Build history of the part. All positions in model axes, mm. Face numbers are marked on the shaded views. A direction names the side the tool comes from. Coordinates: 2 decimals unless noted, no trailing zeros. Loops run counter-clockwise (first coordinate to the right, second up) from the corner with the lowest first, then second, coordinate; pieces in that order, holes last. Notation, with made-up numbers: (53.25, 58.25) - (78.25, 58.25) arc R28 cw to (78.25, 97.25) - close; hole circle Ø5 at (9, 74.25). An arc over 180 degrees is marked (long way). One line per item, written item: value.
```python
from build123d import *

# Parameters (mm, degrees)
SKETCH1_R           = 1.4
BOSS_EXTRUDE1_DEPTH = 8.5


with BuildPart() as part:
    # Sketch1 → Boss-Extrude1 (new body)
    with BuildSketch(Plane(origin=(0, -3.71400402, 0), x_dir=(1, 0, 0), z_dir=(0, 1, 0))):
        with BuildLine():
            ThreePointArc((-114.649243174, 10.730908874), (-116.044111605, 12.812074413), (-118.499243174, 12.312838076))
            Line((-118.499243174, 12.312838076), (-118.499243174, 11.190908874))
            Line((-118.499243174, 11.190908874), (-119.101719053, 11.190908874))
            ThreePointArc((-119.101719053, 11.190908874), (-117.130467384, 8.49282144), (-114.649243174, 10.730908874))
        make_face()
        with Locations((-116.899243174, 10.730908874)):
            Circle(SKETCH1_R, mode=Mode.SUBTRACT)
    extrude(amount=BOSS_EXTRUDE1_DEPTH)


solid = part.part
```
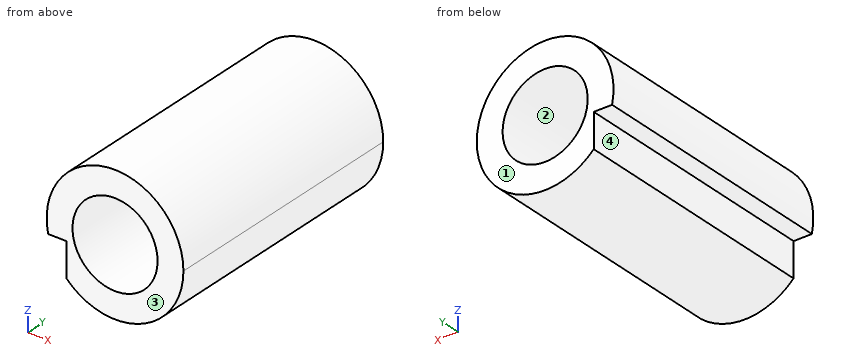
Item 1: Cut at D-D, the plane x = -115.05. Write the cut outline in (y, z).
Check result:
outline: (-3.71, -12.01) - (4.79, -12.01) - (4.79, -9.45) - (-3.71, -9.45) - close
Item 2: Drop flat-ended pins along their axis: P1, Ø0.5, axis at x = -119, y = 1, coming from the -Z side; P2, Ø0.6, axis at y = 1.5, z = -12, coming from the -X side; P3, Ø2, axis at x = -116.9, z = -10.73, coming from the +Y side; P4, Ø1, axis at y = 2, z = -9.5, coming from the -X side. Give the stop position or say it passes through.
Check result:
P1: stops at z = -11.19
P2: stops at x = -118.5
P3: passes through
P4: stops at x = -119.03
Item 3: Cut at A-A, the plane x = -115.8. Write the cut outline in (y, z).
Check result:
outline: (-3.71, -12.69) - (4.79, -12.69) - (4.79, -11.6) - (-3.71, -11.6) - close; (-3.71, -9.86) - (4.79, -9.86) - (4.79, -8.77) - (-3.71, -8.77) - close
Item 4: Pull direction Z, two halves, no side cores. Call the marked faces 1 and 2: released by +Z, released by -Z, zero draft, split by the parting line, or undercut.
Check result:
face 1: zero draft
face 2: undercut
Item 5: Tool access for the marked faces 3 and 4: list every direction of +Z, -Z, +X, -X, +Y, -Y with a clear straight run to the whole face (end or side of a thin tool).
Check result:
face 3: +Z, -Z, +X, -X, -Y
face 4: -Z, -X, +Y, -Y
Item 6: Probe probe 1 along X at (y, z) = (-0.75, -10.75); probe 2 along X at (y, z) = (4.25, -10.25); probe 3 along Z at (x, y) = (-116.4, 1.5). List the from-to ranges inside material, lowest first. Write a range as from..to.
Check result:
probe 1: x = -119.15..-118.3, -115.5..-114.65
probe 2: x = -119.1..-118.21, -115.58..-114.7
probe 3: z = -12.92..-12.04, -9.42..-8.54
Item 7: Cut at B-B, the plane z = -10.4. Write the cut outline in (x, y), then the cut area to 3 significant figures.
Check result:
outline: (-119.12, -3.71) - (-118.26, -3.71) - (-118.26, 4.79) - (-119.12, 4.79) - close; (-115.54, -3.71) - (-114.67, -3.71) - (-114.67, 4.79) - (-115.54, 4.79) - close
area: 14.7 mm^2
Item 8: Cut at C-C, the plane y = 0.25. Write the cut outline in (x, z).
Check result:
outline: (-119.1, -11.19) - (-118.5, -11.19) - (-118.5, -12.31) arc R2.25 ccw (long way) to start; hole circle Ø2.8 at (-116.9, -10.73)
